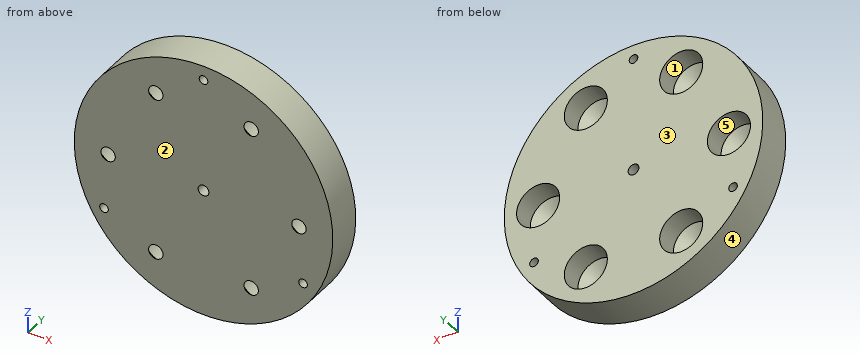
from build123d import *

# Parameters (mm, degrees)
BOSS_EXTRUDE1_DEPTH       = 10.425440853
BOSS_EXTRUDE1_DEPTH_BACK  = 2
SKETCH1_R                 = 45
F_8_0MM_DOWEL_HOLE1_D     = 15
F_8_0MM_DOWEL_HOLE1_DEPTH = 7.425440853
F_8_0MM_DOWEL_HOLE1_TIP   = 7.5
F_3_0_3_DIAMETER_HOLE1_D  = 3
SKETCH2_R                 = 1.875
CUT_EXTRUDE1_DEPTH        = 15


with BuildPart() as part:
    # Sketch1 → Boss-Extrude1 (new, two sides: drawn at the far end of the back side and taken through both)
    with BuildSketch(Plane(origin=(0, 0, 0), x_dir=(1, 0, 0), z_dir=(0, 1, 0)).offset(-BOSS_EXTRUDE1_DEPTH_BACK)):
        with Locations(Location((0, 0, 0), (0, 0, 270))):
            Circle(SKETCH1_R)
    extrude(amount=BOSS_EXTRUDE1_DEPTH + BOSS_EXTRUDE1_DEPTH_BACK)

    # Ø8.0mm Dowel Hole1
    with Locations(Plane(origin=(0, 10.425440853, 0), x_dir=(1, 0, 0), z_dir=(0, 1, 0))):
        with Locations((-16.606971943, 28.764119165), (-16.606971943, -28.764119165), (33.213943886, 0), (16.606971943, 28.764119165), (16.606971943, -28.764119165), (-33.213943886, 0)):
            Hole(F_8_0MM_DOWEL_HOLE1_D / 2, depth=F_8_0MM_DOWEL_HOLE1_DEPTH)
            with Locations((0, 0, -(F_8_0MM_DOWEL_HOLE1_DEPTH + F_8_0MM_DOWEL_HOLE1_TIP / 2))):  # 90° drill point
                Cone(0, F_8_0MM_DOWEL_HOLE1_D / 2, F_8_0MM_DOWEL_HOLE1_TIP, mode=Mode.SUBTRACT)

    # Ø3.0 (3) Diameter Hole1 (through all)
    with Locations(Plane(origin=(0, 10.425440853, 0), x_dir=(1, 0, 0), z_dir=(0, 1, 0))):
        with Locations((-34.641016151, 20), (0, -40), (34.641016151, 20)):
            Hole(F_3_0_3_DIAMETER_HOLE1_D / 2)

    # Sketch2 → Cut-Extrude1 (cut)
    with BuildSketch(Plane(origin=(0, 10.425440853, 0), x_dir=(1, 0, 0), z_dir=(0, 1, 0))):
        with Locations(Location((0, 0, 0), (0, 0, 270))):
            Circle(SKETCH2_R)
    extrude(amount=-CUT_EXTRUDE1_DEPTH, mode=Mode.SUBTRACT)


solid = part.part
The listing builds one solid part. Answer for the finished solid, in the listing's coordinates (mm). Face numbers are marked on the shaded views. A direction names the side the tool comes from. Round coordinates to 2 decimals unless told otherwise and drop trailing zeros. Order: outer loops, then holes, each group sorted by start corner. A loop starts at its lowest first (then second) coordinate and runs counter-clockwise, first axis right, second up. Notation, with made-up numbers: (89.5, 50.25) - (146.5, 50.25) arc R6 cw to (146.5, 55.25) - close; hole circle Ø10 at (84, 66). An arc over 180 degrees is marked (long way). Write item = value, one per line. Start each with the question number.
1) Section A-A, the plane x = 0 is taken. Write down the section's boundary in (y, z) (3 decimals), plus the area to 3 significant figures.
2) Straight lines are drawn through the part: L1, parallel to Z at x = -13, y = 4.25; L2, parallel to X at y = 10.25, z = -20; L3, parallel to Z at x = -15, y = 1.5. For each, find the intervals that lie inside material, in ascending order.
3) For the marked faces 1 and 2, determine the directions among +Z, -Z, +X, -X, +Y, -Y from which every point of the face is accessible in a straight line to the end or side of a thin tool.
4) Given pin 1 (2 mm diameter, centred on y = 6.5, z = -4, fed in from -X); pin 2 (6 mm diameter, centred on y = 6.5, z = 14, fed in from +X); pin 3 (5 mm diameter, centred on x = -7, y = 6, fed in from -Z), each flat-ended and moving along its own axis, determine where each tip first touches the part or whether it passes through.
5) For a pull along X with two mould halves and no side action, classify the marked faces 3, 4 and 5 as released by +X, released by -X, zero draft, split by the parting line, or undercut.
6) Section D-D, the plane z = 0 is taken. Write down the section's boundary in (x, y) (3 decimals).
7) Section C-C, the plane y = 0 is taken. Count the separate pieces of the cut face and the enclosed holes in it, plus the area to 3 significant figures.
8) Section B-B, the plane z = 40 is taken. Write down the section's boundary in (x, y), plus the area to 3 significant figures.
Results list:
q1.outline = (-2, -45) - (10.425, -45) - (10.425, -1.875) - (-2, -1.875) - close; (-2, 1.875) - (10.425, 1.875) - (10.425, 38.5) - (-2, 38.5) - close; (-2, 41.5) - (10.425, 41.5) - (10.425, 45) - (-2, 45) - close
q1.area = 1,030 mm^2
q2.L1 = -43.08 to -35.34, -22.19 to 22.19, 35.34 to 43.08
q2.L2 = -40.31 to -36.14, -33.14 to 33.14, 36.14 to 40.31
q2.L3 = -42.43 to -34.54, -22.98 to 22.98, 34.54 to 42.43
q3.face_1 = +Y
q3.face_2 = +Z, -Z, +X, -X, -Y
q4.pin_1 = -44.9
q4.pin_2 = 43.63
q4.pin_3 = -44.77
q5.face_3 = zero draft
q5.face_4 = split by the parting line
q5.face_5 = undercut
q6.outline = (-45, -2) - (-35.714, -2) - (-40.714, 3) - (-40.714, 10.425) - (-45, 10.425) - close; (-30.714, -2) - (-1.875, -2) - (-1.875, 10.425) - (-25.714, 10.425) - (-25.714, 3) - close; (1.875, -2) - (30.714, -2) - (25.714, 3) - (25.714, 10.425) - (1.875, 10.425) - close; (35.714, -2) - (45, -2) - (45, 10.425) - (40.714, 10.425) - (40.714, 3) - close
q7.separate_pieces = 1
q7.enclosed_holes = 10
q7.area = 5,950 mm^2
q8.outline = (-20.62, -2) - (-1.5, -2) - (-1.5, 10.43) - (-20.62, 10.43) - close; (1.5, -2) - (20.62, -2) - (20.62, 10.43) - (1.5, 10.43) - close
q8.area = 475 mm^2
